Source: CAD feature listing. Evaluate the final solid. Frame: model axes, mm. A direction names the side the tool comes from. Round coordinates to 2 decimals unless told otherwise and drop trailing zeros. Order: outer loops, then holes, each group sorted by start corner. A loop starts at its lowest first (then second) coordinate and runs counter-clockwise, first axis right, second up. Notation, with made-up numbers: (5.5, -6) -> (39.5, -6) arc R10 cw to (39.5, 10) -> close; hole circle Ø10 at (77, 85). An arc over 180 degrees is marked (long way). One line per item, written item: value. Start each with the question number.
1) Reachability of faces 1 (the face through (-19, 5, -3.5)), 2 (the face through (-28.5, 4, -21)), 3 (the face through (-3, 2, -39)) from +Z, -Z, +X, -X, +Y, -Y: full face, straight path, thin tool, end or side. Return the list, or none.
2) Mould query, pull axis Z, two halves, no side actions, for faces 4 (the face through (-3.6, 4.7, -19.2)), 5 (the face through (26.582, 4.056, -4.273)), 6 (the face through (-18.4, 2.2, -39)). Classes: pulls with the +Z half, pulls with the -Z half, needs draft (parallel to the pull), parting line crosses it, or undercut.
3) Section B-B (x = -24.5). Return the cut outline in (y, z).
4) Section D-D (x = 24.5). Return the cut outline in (y, z), and give its area (3 significant figures).
5) Ray query, L1, parallel to X at y = 5, z = -4; L2, parallel to X at y = 6.25, z = -38; L3, parallel to X at y = 3.25, z = -5. Return the intervals inside material, ascending.
6) Section A-A (z = -16). Return the cut outline in (x, y).
7) Pin query (flat end, axial travel): P1, Ø6.5, axis at x = 24.5, z = -4, coming from the +Y side; P2, Ø1.5, axis at x = -3, y = 2, coming from the +Z side; P3, Ø4, axis at x = 24.5, z = -38, coming from the -Y side. Return the tip coordinate at first contact, or that it passes through.
8) Section C-C (y = 7). Return the cut outline in (x, z), and give its area (3 significant figures).
```python
from build123d import *

# Parameters (mm, degrees)
SALIENTE_EXTRUIR1_DEPTH = 42
CROQUIS2_W              = 9.3
CROQUIS2_H              = 28
CORTAR_EXTRUIR1_DEPTH   = 50
CROQUIS3_R              = 2.1
CORTAR_EXTRUIR2_DEPTH   = 50
SALIENTE_EXTRUIR2_START = -3
SALIENTE_EXTRUIR2_DEPTH = 3


with BuildPart() as part:
    # Croquis1 → Saliente-Extruir1 (new body)
    with BuildSketch(Plane.XY):
        with BuildLine():
            Line((-28.5, 8), (-28.5, 0))
            Line((-28.5, 0), (-22.1, 0))
            ThreePointArc((-22.1, 0), (-18.5, 3.6), (-14.9, 0))
            Line((-14.9, 0), (-8.2, 0))
            ThreePointArc((-8.2, 0), (-3.5, 4.7), (1.2, 0))
            Line((1.2, 0), (10.8, 0))
            ThreePointArc((10.8, 0), (15.5, 4.7), (20.2, 0))
            Line((20.2, 0), (28.5, 0))
            Line((28.5, 0), (28.5, 8))
            Line((28.5, 8), (-28.5, 8))
        make_face()
    extrude(amount=-SALIENTE_EXTRUIR1_DEPTH)

    # Croquis2 → Cortar-Extruir1 (cut)
    with BuildSketch(Plane(origin=(0, 8, 0), x_dir=(1, 0, 0), z_dir=(0, 1, 0))):
        with Locations((-18.5, 17.5)):
            Rectangle(CROQUIS2_W, CROQUIS2_H)
    extrude(amount=-CORTAR_EXTRUIR1_DEPTH, mode=Mode.SUBTRACT)

    # Croquis3 → Cortar-Extruir2 (cut)
    with BuildSketch(Plane(origin=(0, 8, 0), x_dir=(1, 0, 0), z_dir=(0, 1, 0))):
        with Locations(Location((-24.5, 38, 0), (0, 0, 270))):
            Circle(CROQUIS3_R)
        with Locations(Location((24.5, 38, 0), (0, 0, 270))):
            Circle(CROQUIS3_R)
        with Locations(Location((24.5, 4, 0), (0, 0, 270))):
            Circle(CROQUIS3_R)
    extrude(amount=-CORTAR_EXTRUIR2_DEPTH, mode=Mode.SUBTRACT)

    # Croquis4 → Saliente-Extruir2 (add)
    with BuildSketch(Plane(origin=(0, 0, -42), x_dir=(-1, 0, 0), z_dir=(0, 0, -1)).offset(SALIENTE_EXTRUIR2_START)):
        with BuildLine():
            ThreePointArc((-10.8, 0), (-15.5, 4.7), (-20.2, 0))
            Line((-20.2, 0), (-17, 0))
            ThreePointArc((-17, 0), (-15.5, 1.5), (-14, 0))
            Line((-14, 0), (-10.8, 0))
        make_face()
        with BuildLine():
            ThreePointArc((8.2, 0), (3.5, 4.7), (-1.2, 0))
            Line((-1.2, 0), (2, 0))
            ThreePointArc((2, 0), (3.5, 1.5), (5, 0))
            Line((5, 0), (8.2, 0))
        make_face()
        with BuildLine():
            ThreePointArc((22.1, 0), (18.5, 3.6), (14.9, 0))
            Line((14.9, 0), (16.5, 0))
            ThreePointArc((16.5, 0), (18.5, 2), (20.5, 0))
            Line((20.5, 0), (22.1, 0))
        make_face()
    extrude(amount=SALIENTE_EXTRUIR2_DEPTH)


solid = part.part
```
Findings:
1. face 1: +Y, -Y
1. face 2: +Z, -Z, -X, +Y, -Y
1. face 3: +Z, -Y
2. face 4: needs draft
2. face 5: undercut
2. face 6: pulls with the +Z half
3. outline: (0, -42) -> (8, -42) -> (8, -40.1) -> (0, -40.1) -> close; (0, -35.9) -> (8, -35.9) -> (8, 0) -> (0, 0) -> close
4. outline: (0, -42) -> (8, -42) -> (8, -40.1) -> (0, -40.1) -> close; (0, -35.9) -> (8, -35.9) -> (8, -6.1) -> (0, -6.1) -> close; (0, -1.9) -> (8, -1.9) -> (8, 0) -> (0, 0) -> close
4. area: 269 mm2
5. L1: -28.5 to -23.15, -13.85 to 22.4, 26.6 to 28.5
5. L2: -28.5 to -26.6, -22.4 to 22.4, 26.6 to 28.5
5. L3: -28.5 to -23.15, -13.85 to -6.9, -0.1 to 12.1, 18.9 to 22.65, 26.35 to 28.5
6. outline: (-28.5, 0) -> (-23.15, 0) -> (-23.15, 8) -> (-28.5, 8) -> close; (-13.85, 0) -> (-8.2, 0) arc R4.7 cw to (1.2, 0) -> (10.8, 0) arc R4.7 cw to (20.2, 0) -> (28.5, 0) -> (28.5, 8) -> (-13.85, 8) -> close
7. P1: y = 8
7. P2: z = -39
7. P3: through
8. outline: (-28.5, -42) -> (28.5, -42) -> (28.5, 0) -> (-28.5, 0) -> close; hole circle Ø4.2 at (-24.5, -38); hole (-23.15, -31.5) -> (-13.85, -31.5) -> (-13.85, -3.5) -> (-23.15, -3.5) -> close; hole circle Ø4.2 at (24.5, -38); hole circle Ø4.2 at (24.5, -4)
8. area: 2,090 mm2
